Can you work these out from the drawing? Everything is in mm from the part's minimum corner. Coordinates: 2 decimals unless noted, no trailing zeros. Loops run counter-clockwise (first coordinate to the right, second up) from the corner with the lowest first, then second, coordinate; pieces in that order, holes last.
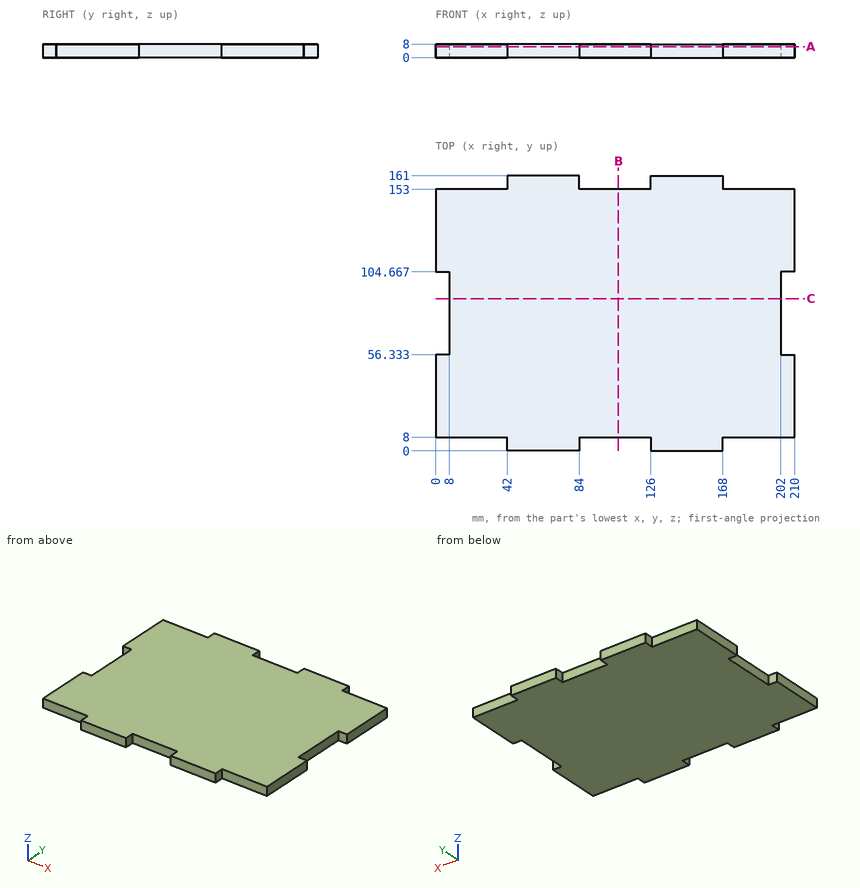
Item 1: Suppose I cut it at A-A, the plane z = 6.5. Please give me the cut outline in (x, y), plus the area to 3 significant figures.
Results are:
outline: (0, 8) - (42, 8) - (42, 0) - (84, 0) - (84, 8) - (126, 8) - (126, 0) - (168, 0) - (168, 8) - (210, 8) - (210, 56.33) - (202, 56.33) - (202, 104.67) - (210, 104.67) - (210, 153) - (168, 153) - (168, 161) - (126, 161) - (126, 153) - (84, 153) - (84, 161) - (42, 161) - (42, 153) - (0, 153) - (0, 104.67) - (8, 104.67) - (8, 56.33) - (0, 56.33) - close
area: 31,000 mm2
Item 2: Suppose I cut it at C-C, the plane y = 89. Please give me the cut outline in (x, z), plus the area to 3 significant figures.
Results are:
outline: (8, 0) - (202, 0) - (202, 8) - (8, 8) - close
area: 1,550 mm2
Item 3: Suppose I cut it at B-B, the plane x = 107. Please give me the cut outline in (y, z), plus the area to 3 significant figures.
Results are:
outline: (8, 0) - (153, 0) - (153, 8) - (8, 8) - close
area: 1,160 mm2
Item 4: I'm going to push flat-ended pins straight in: P1, Ø4, axis at x = 22, z = 4, coming from the -Y side; P2, Ø3, axis at x = 28, z = 1.5, coming from the +Y side; P3, Ø2, axis at y = 24, z = 3, coming from the -X side; P4, Ø4, axis at y = 158.5, z = 3.5, coming from the -X side. Where does each tip first touch, or does it pass through?
Results are:
P1: stops at y = 8
P2: stops at y = 153
P3: stops at x = 0
P4: stops at x = 42
Item 5: I need wall thicknesses on line 1 along X through (y, z) = (154, 4.75); line 2 along Y through (x, z) = (34, 5.25); line 3 along X through (y, z) = (78, 1.25). Which ranges of each line are inside material? Lowest first, please.
Results are:
line 1: x = 42 to 84, 126 to 168
line 2: y = 8 to 153
line 3: x = 8 to 202
